```python
from build123d import *

# Parameters (mm, degrees)
FILLET1_R          = 5
CUT_EXTRUDE1_START = -3
CUT_EXTRUDE1_DEPTH = 3
SKETCH4_R          = 7.925
CUT_EXTRUDE2_DEPTH = 20


with BuildPart() as part:
    # Sketch2 → Revolve1 (revolve)
    with BuildSketch(Plane.XY, mode=Mode.PRIVATE) as revolve1_sk:
        Polygon((15.075, -67.5), (0, -67.5), (0, 67.5), (1, 67.5), (1, 35.6), (2.825, 33.749724479), (2.825, 22), (5.275, 22), (5.275, 13.9), (9.4, 13.9), (9.4, -64.5), (15.075, -64.5), align=None)
    revolve(revolve1_sk.sketch.rotate(Axis((0, 24.52235385, 0), (0, -1, 0)), 90), axis=Axis((0, 24.52235385, 0), (0, -1, 0)))

    # Fillet1
    # the kernel refuses this fillet: 5 mm, written as the material it takes off along each edge
    with BuildSketch(Plane(origin=(0, 13.9, 0), x_dir=(0, 0, 1), z_dir=(1, 0, 0))) as fillet1_piece_1:
        with BuildLine():
            CenterArc((4.4, 4.922842167), FILLET1_R, 280.078658108, 79.921341892)
            Line((9.4, 4.922842167), (9.5, 4.922842167))
            Line((9.5, 4.922842167), (9.5, 0))
            Line((9.5, 0), (9.4, -0.1))
            ThreePointArc((9.4, -0.1), (7.3375, -0.1), (5.2925, -0.098456843))
            Line((5.2925, -0.098456843), (5.275, 0))
        make_face()
    revolve(axis=Axis((0, 13.9, 0), (0, -1, 0)), mode=Mode.SUBTRACT)

    # Sketch3 → Cut-Extrude1 (cut)
    with BuildSketch(Plane(origin=(0, -64.5, 0), x_dir=(1, 0, 0), z_dir=(0, 1, 0)).offset(CUT_EXTRUDE1_START)):
        with BuildLine():
            Line((-12.854571171, 7.875), (-8.20822758, 7.875))
            ThreePointArc((-8.20822758, 7.875), (0, 11.375), (8.20822758, 7.875))
            Line((8.20822758, 7.875), (12.854571171, 7.875))
            ThreePointArc((12.854571171, 7.875), (0, 15.075), (-12.854571171, 7.875))
        make_face()
        with BuildLine():
            Line((-12.854571171, -7.875), (-8.20822758, -7.875))
            ThreePointArc((-8.20822758, -7.875), (0, -11.375), (8.20822758, -7.875))
            Line((8.20822758, -7.875), (12.854571171, -7.875))
            ThreePointArc((12.854571171, -7.875), (0, -15.075), (-12.854571171, -7.875))
        make_face()
    extrude(amount=CUT_EXTRUDE1_DEPTH, mode=Mode.SUBTRACT)

    # Sketch4 → Cut-Extrude2 (cut)
    with BuildSketch(Plane.XZ.offset(67.5)):
        with Locations(Location((0, 0, 0), (0, 0, 270))):
            Circle(SKETCH4_R)
    extrude(amount=-CUT_EXTRUDE2_DEPTH, mode=Mode.SUBTRACT)


solid = part.part
```
Check sheet for the modelled part. Datum: model origin and axes. Units: mm. A direction names the side the tool comes from. Give positions to 0.01 mm unless a question says otherwise; leave off trailing zeros. Write each loop counter-clockwise with the first axis right and the second up, starting at its lowest first coordinate (ties: lowest second). Pieces come first, ordered by that corner, then holes.
Item 1: Cross-section at A-A (y = -51.5). Enter the section's corners in (x, z) (3 decimals), and give its area (3 significant figures).
Item 2: Access from +Z, -Z, +X, -X, +Y, -Y to the whole of each face (thin tool, end or side, straight path). Record for faces 5 (the face through (-11, -66, -7.875)), 6 (the face through (-11, -66, 7.875)), 7 (the face through (-0.849, 27.793, 2.695)).
Item 3: Draft check along X on faces 1 (the face through (-4.82, -57.64, 6.29)), 2 (the face through (-1.584, 17.893, 5.031)), 3 (the face through (0, -47.5, 0)), 4 (the face through (2.3, 22, -2.3)). Enter one of: released by +X, released by -X, zero draft, split by the parting line, or undercut.
Item 4: Scan lines: L1, parallel to X at y = -60.75, z = 0 (3 decimals); L2, parallel to Z at x = 0, y = -16.5; L3, parallel to X at y = -57, z = 2.75. Record each from-to range of solid material in increasing order.
Item 5: Gauge pin test, flat ends, axial feed: pin 1 (8.5 mm diameter, centred on x = -1, z = 1, fed in from +Y); pin 2 (10 mm diameter, centred on y = 40.5, z = 1.5, fed in from -X); pin 3 (2.5 mm diameter, centred on x = -10.5, y = -65.5, fed in from +Z) (3 decimals); pin 4 (3.5 mm diameter, centred on x = 10, y = -66.5, fed in from -Z) (3 decimals). Record the tip position at first contact, or that the pin passes through.
Report:
1. outline: circle Ø18.8 at (0, 0); hole circle Ø15.85 at (0, 0)
1. area: 80.3 mm2
2. face 5: -Z, -X, +Y, -Y
2. face 6: +Z, -X, +Y, -Y
2. face 7: +Y
3. face 1: undercut
3. face 2: split by the parting line
3. face 3: undercut
3. face 4: zero draft
4. L1: x = -9.4 to -7.925, 7.925 to 9.4
4. L2: z = -9.4 to 9.4
4. L3: x = -8.99 to -7.43, 7.43 to 8.99
5. pin 1: stops at y = 67.5
5. pin 2: stops at x = -1
5. pin 3: stops at z = 7.875
5. pin 4: stops at z = -7.875
